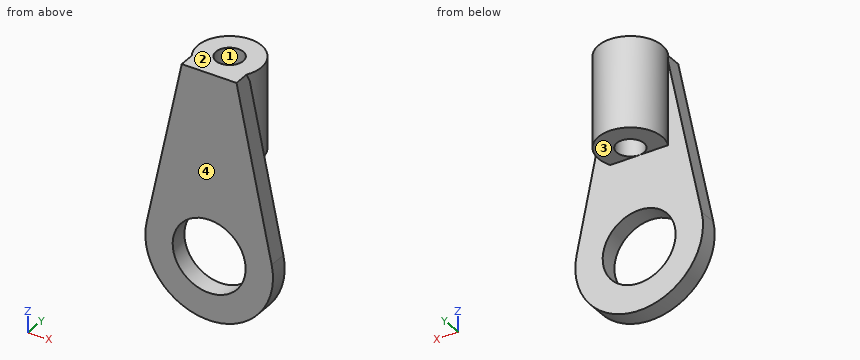
from build123d import *

# Parameters (mm, degrees)
SKETCH_1_R          = 2
EXTRUDE_1_DEPTH     = 1
EXTRUDE_START       = 10
SKETCH_2_R          = 1.75
EXTRUDE_2_DEPTH     = 5
SKETCH_3_R          = 0.75
CUT_EXTRUDE_1_DEPTH = 5


with BuildPart() as part:
    # 草图1 → 凸台-拉伸1 (new body)
    with BuildSketch(Plane(origin=(0, 0, 0), x_dir=(1, 0, 0), z_dir=(0, 1, 0))):
        with BuildLine():
            Line((-1.5, -10), (1.5, -10))
            Line((1.5, -10), (3.427033294, -0.710945006))
            ThreePointArc((3.427033294, -0.710945006), (0, 3.5), (-3.427033294, -0.710945006))
            Line((-3.427033294, -0.710945006), (-1.5, -10))
        make_face()
        with Locations(Location((0, 0, 0), (0, 0, 270))):
            Circle(SKETCH_1_R, mode=Mode.SUBTRACT)
    extrude(amount=EXTRUDE_1_DEPTH)

    # 草图2 → 凸台-拉伸2 (add)
    with BuildSketch(Plane.XY.offset(EXTRUDE_START)):
        with Locations((0, 1.75)):
            Circle(SKETCH_2_R)
    extrude(amount=-EXTRUDE_2_DEPTH)

    # 草图3 → 切除-拉伸1 (cut)
    with BuildSketch(Plane(origin=(0, 0, 5), x_dir=(-1, 0, 0), z_dir=(0, 0, -1))):
        with Locations((0, 1.75)):
            Circle(SKETCH_3_R)
    extrude(amount=-CUT_EXTRUDE_1_DEPTH, mode=Mode.SUBTRACT)


solid = part.part
Model file for the job. Use its own axes, mm. Face numbers are marked on the shaded views. A direction names the side the tool comes from. Round coordinates to 2 decimals unless told otherwise and drop trailing zeros. Loops run counter-clockwise (first coordinate to the right, second up) from the corner with the lowest first, then second, coordinate; pieces in that order, holes last. Notation, with made-up numbers: (9, -4.5) -> (65, -4.5) arc R27 cw to (65, 19.5) -> close; hole circle Ø10 at (-11.75, 10.5). An arc over 180 degrees is marked (long way). Answer as CSV lines item,"result". Start each with the question number.
1) Probe line 1 along X through (y, z) = (0.35, 0); line 2 along Y through (x, z) = (0, 8.25); line 3 along X through (y, z) = (1.75, 7.55). List the from-to ranges inside material, lowest first.
2) Slice it at B-B (y = 1.75). List the corners of the cut face in (x, z), plus the area to 3 significant figures.
3) Pin check, flat tips, straight feed: P1, Ø1, axis at x = -2.5, z = -2, coming from the +Y side; P2, Ø1.5, axis at x = 0, y = 3, coming from the -Z side; P3, Ø2, axis at y = 1, z = -1, coming from the -X side; P4, Ø1.2, axis at x = 0, y = 1.75, coming from the +Z side. Stop position of each tip, or through.
4) Mould opens along X. For the marked faces 1 and 2 say: +X half, -X half, draft (parallel to the pull), parting line (faces both ways), or undercut.
5) Tool access for the marked faces 3 and 4: list every direction of +Z, -Z, +X, -X, +Y, -Y with a clear straight run to the whole face (end or side of a thin tool).
6) Slice it at D-D (z = 6.5). List the corners of the cut face in (x, y), plus the area to 3 significant figures.
7) Slice it at A-A (z = 0). List the corners of the cut face in (x, y), plus the area to 3 significant figures.
8) Slice it at C-C (x = 0.5). List the corners of the cut face in (y, z).
Filled in:
1,line 1,"x = -3.5 to -2, 2 to 3.5"
1,line 2,"y = 0 to 1, 2.5 to 3.5"
1,line 3,"x = -1.75 to -0.75, 0.75 to 1.75"
2,outline,"(-1.75, 5) -> (-0.75, 5) -> (-0.75, 10) -> (-1.75, 10) -> close; (0.75, 5) -> (1.75, 5) -> (1.75, 10) -> (0.75, 10) -> close"
2,area,"10.0 mm2"
3,P1,"stops at y = 1"
3,P2,"stops at z = 5"
3,P3,"stops at x = -3.5"
3,P4,"passes through"
4,face 1,"undercut"
4,face 2,"draft"
5,face 3,"-Z, +X, -X, +Y"
5,face 4,"+Z, -Z, +X, -X, -Y"
6,outline,"(-2.23, 0) -> (2.23, 0) -> (2.23, 1) -> (1.58, 1) arc R1.75 ccw (long way) to (-1.58, 1) -> (-2.23, 1) -> close; hole circle Ø1.5 at (0, 1.75)"
6,area,"10.0 mm2"
7,outline,"(-3.5, 0) -> (-2, 0) -> (-2, 1) -> (-3.5, 1) -> close; (2, 0) -> (3.5, 0) -> (3.5, 1) -> (2, 1) -> close"
7,area,"3.00 mm2"
8,outline,"(0, -3.46) -> (1, -3.46) -> (1, -1.94) -> (0, -1.94) -> close; (0, 1.94) -> (1, 1.94) -> (1, 5) -> (1.19, 5) -> (1.19, 10) -> (0, 10) -> close; (2.31, 5) -> (3.43, 5) -> (3.43, 10) -> (2.31, 10) -> close"
